```python
from build123d import *

# Parameters (mm, degrees)
SKETCH1_W                                  = 50
SKETCH1_H                                  = 50
BOSS_EXTRUDE1_DEPTH                        = 30
SKETCH3_R                                  = 6
CUT_EXTRUDE1_DEPTH                         = 70
SKETCH5_W                                  = 41
SKETCH5_H                                  = 51
CUT_EXTRUDE3_DEPTH                         = 48
SKETCH7_R                                  = 1.75
CUT_EXTRUDE5_DEPTH                         = 60
CIRPATTERN3_COUNT                          = 3
SKETCH8_W                                  = 2
SKETCH8_H                                  = 3
CUT_EXTRUDE6_DEPTH                         = 60
MIRROR1_AT_THE_SECOND_PLANE_COPY_1_SKETC_W = 2
MIRROR1_AT_THE_SECOND_PLANE_COPY_1_SKETC_H = 3
MIRROR1_AT_THE_SECOND_PLANE_COPY_1_DEPTH   = 60
SKETCH9_W                                  = 40
SKETCH9_H                                  = 5
CUT_EXTRUDE7_DEPTH                         = 40
SKETCH10_R                                 = 3.5
CUT_EXTRUDE8_DEPTH                         = 2.5
CIRPATTERN4_COUNT                          = 3
MIRROR2_COPY_1_SKETCH_R                    = 3.5
MIRROR2_COPY_1_DEPTH                       = 2.5
MIRROR2_COPY_2_SKETCH_R                    = 3.5
MIRROR2_COPY_2_DEPTH                       = 2.5


with BuildPart() as part:
    # Sketch1 → Boss-Extrude1 (new, symmetric)
    with BuildSketch(Plane.XY):
        Rectangle(SKETCH1_W, SKETCH1_H)
    extrude(amount=BOSS_EXTRUDE1_DEPTH, both=True)

    # Sketch3 → Cut-Extrude1 (cut)
    with BuildSketch(Plane.XY.offset(30)):
        Circle(SKETCH3_R)
    extrude(amount=-CUT_EXTRUDE1_DEPTH, mode=Mode.SUBTRACT)

    # Sketch5 → Cut-Extrude3 (cut)
    with BuildSketch(Plane(origin=(0, 25, 0), x_dir=(1, 0, 0), z_dir=(0, 1, 0))):
        Rectangle(SKETCH5_W, SKETCH5_H)
    extrude(amount=-CUT_EXTRUDE3_DEPTH, mode=Mode.SUBTRACT)

    # Sketch7 → Cut-Extrude5 (cut)
    with BuildSketch(Plane.XY.offset(30)):
        with Locations((0, 12)):
            Circle(SKETCH7_R)
    cut_extrude5 = extrude(amount=-CUT_EXTRUDE5_DEPTH, mode=Mode.SUBTRACT)

    # CirPattern3: Cut-Extrude5 ×3 about axis
    cirpattern3_axis = Axis((0, 0, 0), (0, 0, 1))
    for i in range(1, CIRPATTERN3_COUNT):
        add(cut_extrude5.rotate(cirpattern3_axis, i * 360 / CIRPATTERN3_COUNT), mode=Mode.SUBTRACT)

    # Sketch8 → Cut-Extrude6 (cut)
    with BuildSketch(Plane.XY.offset(30)):
        with Locations((19, 9)):
            Rectangle(SKETCH8_W, SKETCH8_H)
    cut_extrude6 = extrude(amount=-CUT_EXTRUDE6_DEPTH, mode=Mode.SUBTRACT)

    # Mirror1: Cut-Extrude6 across plane
    add(cut_extrude6.mirror(Plane.ZX), mode=Mode.SUBTRACT)

    # Mirror1 at the second plane: Cut-Extrude6 across plane
    add(cut_extrude6.mirror(Plane(origin=(0, 0, 0), x_dir=(0, 0, 1), z_dir=(1, 0, 0))), mode=Mode.SUBTRACT)

    # Mirror1 at the second plane copy 1 sketc → Mirror1 at the second plane copy 1 (cut)
    with BuildSketch(Plane(origin=(0, 0, 30), x_dir=(-1, 0, 0), z_dir=(0, 0, 1))):
        with Locations((19, 9)):
            Rectangle(MIRROR1_AT_THE_SECOND_PLANE_COPY_1_SKETC_W, MIRROR1_AT_THE_SECOND_PLANE_COPY_1_SKETC_H)
    extrude(amount=-MIRROR1_AT_THE_SECOND_PLANE_COPY_1_DEPTH, mode=Mode.SUBTRACT)

    # Sketch9 → Cut-Extrude7 (cut)
    with BuildSketch(Plane(origin=(25, 0, 0), x_dir=(0, 0, -1), z_dir=(1, 0, 0))):
        with Locations((0, 2)):
            Rectangle(SKETCH9_W, SKETCH9_H)
    extrude(amount=-CUT_EXTRUDE7_DEPTH, mode=Mode.SUBTRACT)

    # Sketch10 → Cut-Extrude8 (cut)
    with BuildSketch(Plane.XY.offset(30)):
        with Locations((0, 12)):
            Circle(SKETCH10_R)
    cut_extrude8 = extrude(amount=-CUT_EXTRUDE8_DEPTH, mode=Mode.SUBTRACT)

    # CirPattern4: Cut-Extrude8 ×3 about axis
    cirpattern4_axis = Axis((0, 0, 0), (0, 0, 1))
    for i in range(1, CIRPATTERN4_COUNT):
        add(cut_extrude8.rotate(cirpattern4_axis, i * 360 / CIRPATTERN4_COUNT), mode=Mode.SUBTRACT)

    # Mirror2: Cut-Extrude8 across plane
    add(cut_extrude8.mirror(Plane.XY), mode=Mode.SUBTRACT)

    # Mirror2 copy 1 sketch → Mirror2 copy 1 (cut)
    with BuildSketch(Plane(origin=(0, 0, -30), x_dir=(-0.4999999999999998, 0.8660254037844387, 0), z_dir=(0, 0, -1))):
        with Locations((0, -12)):
            Circle(MIRROR2_COPY_1_SKETCH_R)
    extrude(amount=-MIRROR2_COPY_1_DEPTH, mode=Mode.SUBTRACT)

    # Mirror2 copy 2 sketch → Mirror2 copy 2 (cut)
    with BuildSketch(Plane(origin=(0, 0, -30), x_dir=(-0.5000000000000004, -0.8660254037844384, 0), z_dir=(0, 0, -1))):
        with Locations((0, -12)):
            Circle(MIRROR2_COPY_2_SKETCH_R)
    extrude(amount=-MIRROR2_COPY_2_DEPTH, mode=Mode.SUBTRACT)


solid = part.part
```
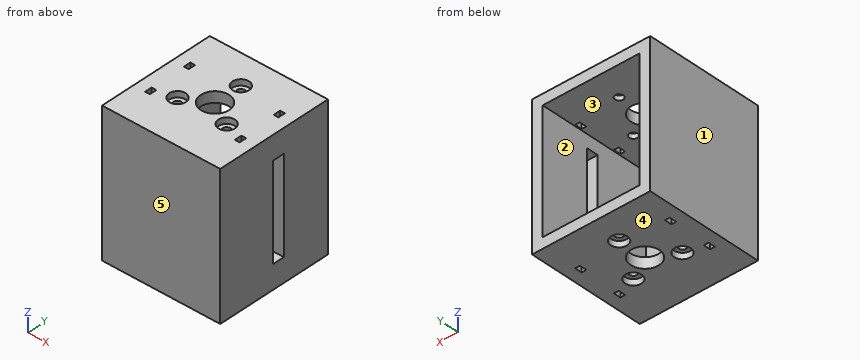
Source: CAD feature listing. Evaluate the final solid. Frame: model axes, mm. Face numbers are marked on the shaded views. A direction names the side the tool comes from. Give positions to 0.01 mm unless a question says otherwise; leave off trailing zeros. Write each loop counter-clockwise with the first axis right and the second up, starting at its lowest first coordinate (ties: lowest second). Pieces come first, ordered by that corner, then holes.
1. Section query C-C (z = -5.5). Return the cut outline in (x, y).
2. Pull-direction query (Z, two-part tool) for the marked faces 3, 4 and 5; classes: +Z half, -Z half, draft (parallel to the pull), parting line (faces both ways), or undercut.
3. First-contact query: pin 1 (2 mm diameter, centred on x = -10.5, y = -6, fed in from +Z); pin 2 (1 mm diameter, centred on x = 9, z = 17, fed in from +Y); pin 3 (2 mm diameter, centred on x = -0.5, y = 10.5, fed in from +Z). Flat tips, straight axial feed; report the tip coordinate or a pass-through.
4. Section query A-A (x = 0). Count the separate pieces of the cut face and the enclosed holes in it, then the cut area to 3 significant figures.
5. Material intervals for line 1 along Y through (x, z) = (0, -26.55); line 2 along X through (y, z) = (22.5, -18); line 3 along Z through (x, y) = (-11, -15), sorted ascending.
6. Section query B-B (y = 18). Return the cut outline in (x, z).
7. Section query D-D (y = 12). Return the cut outline in (x, z).
8. Access query for the marked faces 1 and 2. Directions: +Z, -Z, +X, -X, +Y, -Y. A direction counts if a zero-diameter tool reaches every point of the face in a straight line with its end or side. Return the directions, or none.
Output values:
1. outline: (-25, -25) - (25, -25) - (25, -0.5) - (20.5, -0.5) - (20.5, -23) - (-20.5, -23) - (-20.5, 25) - (-25, 25) - close; (20.5, 4.5) - (25, 4.5) - (25, 25) - (20.5, 25) - close
2. face 3: undercut
2. face 4: -Z half
2. face 5: draft
3. pin 1: passes through
3. pin 2: stops at y = -23
3. pin 3: stops at z = 27.5
4. separate pieces: 5
4. enclosed holes: 0
4. area: 395 mm2
5. line 1: y = -25 to -6, 6 to 10.25, 13.75 to 25
5. line 2: x = -25 to -20.5, 20.5 to 25
5. line 3: z = -30 to -25.5, 25.5 to 30
6. outline: (-25, -30) - (25, -30) - (25, 30) - (-25, 30) - close; hole (-20.5, -25.5) - (20.5, -25.5) - (20.5, 25.5) - (-20.5, 25.5) - close
7. outline: (-25, -30) - (-3.5, -30) - (-3.5, -27.5) - (-1.75, -27.5) - (-1.75, -25.5) - (-20.5, -25.5) - (-20.5, 25.5) - (-1.75, 25.5) - (-1.75, 27.5) - (-3.5, 27.5) - (-3.5, 30) - (-25, 30) - close; (1.75, -27.5) - (3.5, -27.5) - (3.5, -30) - (25, -30) - (25, 30) - (3.5, 30) - (3.5, 27.5) - (1.75, 27.5) - (1.75, 25.5) - (20.5, 25.5) - (20.5, -25.5) - (1.75, -25.5) - close
8. face 1: +Z, -Z, -X, +Y, -Y
8. face 2: +Y
